```python
from build123d import *

# Parameters (mm, degrees)
F0_W     = 76.2
F0_H     = 79.375
F1_DEPTH = 3.175
F2_W     = 19.05
F2_H     = 3.175
F3_DEPTH = 3.176
F4_W     = 3.175
F4_H     = 9.525
F5_DEPTH = 3.176


with BuildPart() as f1:
    # F0 (on Top) → F1 (new body)
    with BuildSketch(Plane.XY):
        Rectangle(F0_W, F0_H)
    extrude(amount=F1_DEPTH)

    # F2 (on face) → F3 (cut, through all)
    with BuildSketch(Plane.XY.offset(3.175)):
        with Locations((-15.875, 38.1)):
            Rectangle(F2_W, F2_H)
        with Locations((15.875, 38.1)):
            Rectangle(F2_W, F2_H)
        with Locations((15.875, -38.1)):
            Rectangle(F2_W, F2_H)
        with Locations((-15.875, -38.1)):
            Rectangle(F2_W, F2_H)
    extrude(amount=-F3_DEPTH, mode=Mode.SUBTRACT)

    # F4 (on face) → F5 (cut, through all)
    with BuildSketch(Plane.XY.offset(3.175)):
        with Locations((-36.5125, 22.225)):
            Rectangle(F4_W, F4_H)
        with Locations((-36.5125, 0)):
            Rectangle(F4_W, F4_H)
        with Locations((-36.5125, -22.225)):
            Rectangle(F4_W, F4_H)
        with Locations((36.5125, -22.225)):
            Rectangle(F4_W, F4_H)
        with Locations((36.5125, 0)):
            Rectangle(F4_W, F4_H)
        with Locations((36.5125, 22.225)):
            Rectangle(F4_W, F4_H)
    extrude(amount=-F5_DEPTH, mode=Mode.SUBTRACT)


solid = f1.part
```
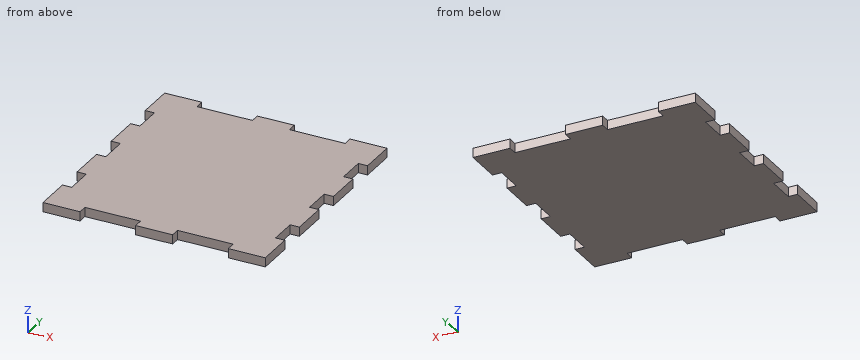
Could you check a few things on this model? Use its own coordinates, in mm. Round coordinates to 2 decimals unless told otherwise and drop trailing zeros. Loops run counter-clockwise (first coordinate to the right, second up) from the corner with the lowest first, then second, coordinate; pieces in that order, holes last. Notation, with made-up numbers: M 19.5,-35.5 L 42.5,-35.5 A3 ccw 42.5,-30.5 Z; hole C 16,29 d2. An arc over 180 degrees is marked long. Put each result on its own line as item: value.
Q1. Imagine slicing it at A-A (x = 9). Write out the boundary of the cut face in (y, z) (1 decimal).
Check result:
outline: M -36.5,0 L 36.5,0 L 36.5,3.2 L -36.5,3.2 Z
Q2. Imagine slicing it at B-B (y = -1). Write out the boundary of the cut face in (x, z) (3 decimals), then the cut area to 3 significant figures.
Check result:
outline: M -34.925,0 L 34.925,0 L 34.925,3.175 L -34.925,3.175 Z
area: 222 mm2
Q3. I need wall thicknesses on probe 1 along Y at (x, z) = (9, 2.85); probe 2 along X at (y, z) = (-4, 0.8) (3 decimals). Which ranges of each line are inside material? Lowest first, please.
Check result:
probe 1: -36.51 to 36.51
probe 2: -34.925 to 34.925
Q4. For pin 1 (1.6 mm diameter, centred on x = -19, z = 2.5, fed in from +Y), with a flat end and sliding along its axis, tell me the tip position at first contact or that it passes through.
Check result:
pin 1: y = 36.51
